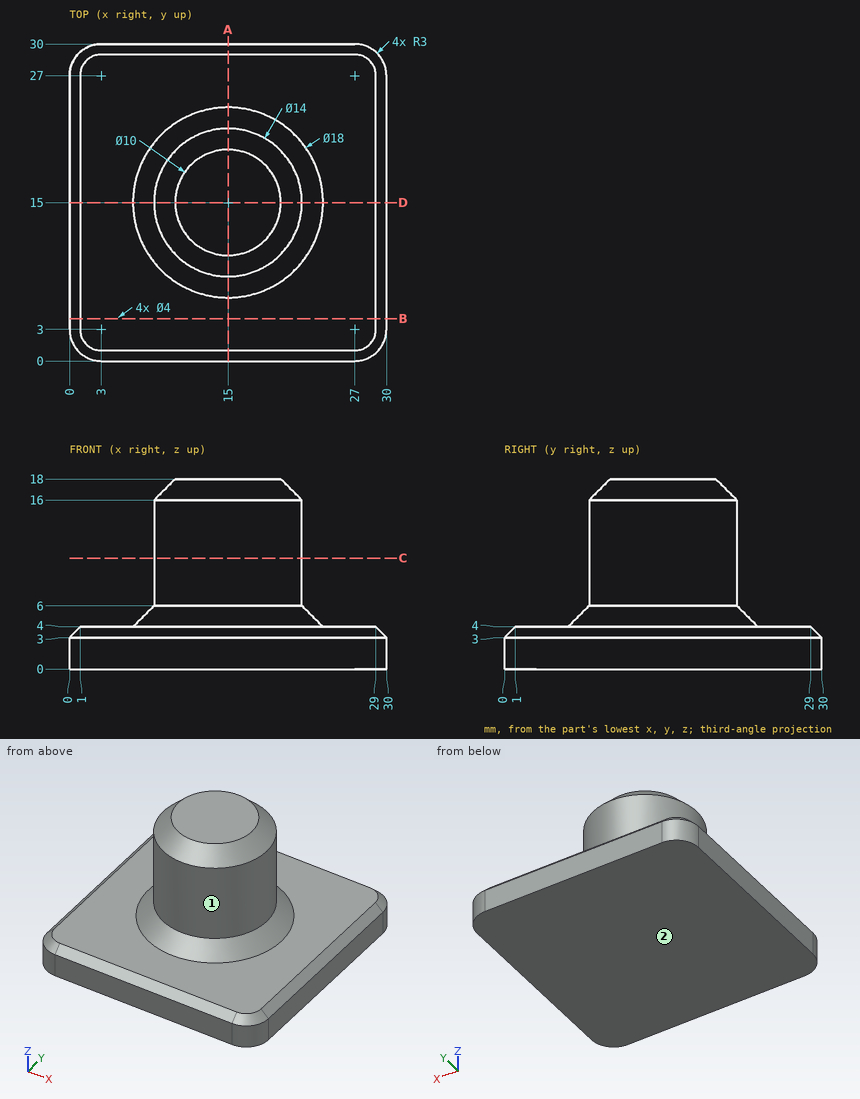
Drawing for the job (mm, zero at the part's lowest x, y, z). A direction names the side the tool comes from. Coordinates: 2 decimals unless noted, no trailing zeros. Loops run counter-clockwise (first coordinate to the right, second up) from the corner with the lowest first, then second, coordinate; pieces in that order, holes last. Notation, with made-up numbers: (-13.5, -35) - (13.5, -35) arc R6 cw to (13.5, -24) - close; hole circle Ø6 at (79.5, 31). An arc over 180 degrees is marked (long way). Return JSON: item names as keys, results as strings.
1. Band-saw the part on C-C (z = 10.5). Give the cut face in (x, y), and give its area (3 significant figures).
Result:
{"outline": "circle Ø14 at (15, 15)", "area": "154 mm2"}
2. Band-saw the part on A-A (x = 15). Give the cut face in (y, z).
Result:
{"outline": "(0, 0) - (30, 0) - (30, 3) - (29, 4) - (24, 4) - (22, 6) - (22, 16) - (20, 18) - (10, 18) - (8, 16) - (8, 6) - (6, 4) - (1, 4) - (0, 3) - close"}
3. Band-saw the part on B-B (y = 4). Give the cut face in (x, z), and give its area (3 significant figures).
Result:
{"outline": "(0, 0) - (30, 0) - (30, 3) - (29, 4) - (1, 4) - (0, 3) - close", "area": "119 mm2"}
4. 3-axis set-ups, long thin cutter, end or side, ignore diameter. For the marked faces 1 and 2: which of +Z, -Z, +X, -X, +Y, -Y reach the whole face in a straight line?
Result:
{"face 1": "+Z", "face 2": "-Z, +X, -X, +Y, -Y"}
5. Drop flat-ended pins along their axis: pin 1 (10 mm diameter, centred on y = 6.5, z = 11.5, fed in from -X); pin 2 (2 mm diameter, centred on x = 13.5, z = 6.5, fed in from -Y); pin 3 (4 mm diameter, centred on x = 7, z = 8, fed in from +Y). Give the stop position or say it passes through.
Result:
{"pin 1": "stops at x = 8.94", "pin 2": "stops at y = 7.63", "pin 3": "stops at y = 18.61"}
6. Probe L1, parallel to Z at x = 28.25, y = 3.25; L2, parallel to Y at x = 19.75, z = 11.5; L3, parallel to Y at x = 16, z = 8.25. List the from-to ranges inside material, lowest first. Write a range as from..to.
Result:
{"L1": "z = 0..4", "L2": "y = 9.86..20.14", "L3": "y = 8.07..21.93"}
